Autodesk Inventor part; units mm, degrees
ref_plane "YZ Plane" through (0, 0, 0) normal (1, 0, 0) x (0, 1, 0)
ref_plane "XZ Plane" through (0, 0, 0) normal (0, 1, 0) x (-1, 0, 0)
ref_plane "XY Plane" through (0, 0, 0) normal (0, 0, 1) x (1, 0, 0)
sketch "Sketch1" plane through (0, 0, 0) normal (0, 1, 0) x (-1, 0, 0)
  arc A0 (0, -177) -> (0, 177) centre (0, 0) ccw
  arc A1 (0, 177) -> (0, -177) centre (0, 0) ccw
  point P0 (-177, 177)
  point P1 (-177, -177)
  dimension "d0" = 354
extrude "Extrusion1" add sketch "Sketch1" along normal blind 5
sketch "Sketch2" plane through (0, 5, 0) normal (0, 1, 0) x (1, 0, 0)
  circle A0 centre (-51.435, -34.125) radius 1.7
  circle A1 centre (-51.435, 34.125) radius 1.7
  circle A2 centre (51.435, 34.125) radius 1.7
  circle A3 centre (51.435, -34.125) radius 1.7
  line L0 (151.6, 177) -> (0, 177) construction
  line L1 (0, -177) -> (0, 177) construction
  circle A4 centre (0, 0) radius 177 construction
  line L2 (-177, 0) -> (177, 0) construction
  circle A5 centre (26.035, 59.5249) radius 1.7
  circle A6 centre (26.035, -59.5249) radius 1.7
  circle A7 centre (-26.035, 59.5249) radius 1.7
  circle A8 centre (-26.035, -59.5249) radius 1.7
  point P0 (177, 177)
  dimension "d5" = 3.4
  dimension "d6" = 3.4
  dimension "d8" = 3.4
  dimension "d10" = 3.4
  dimension "d12" = 68.25
  dimension "d13" = 68.25
  dimension "d14" = 102.87
  dimension "d15" = 102.87
  dimension "d18" = 51.435
  dimension "d19" = 51.435
  dimension "d20" = 34.125
  dimension "d21" = 34.125
  dimension "d153" = 3.4
  dimension "d155" = 3.4
  dimension "d157" = 3.4
  dimension "d159" = 3.4
  dimension "d161" = 52.07
  dimension "d162" = 26.035
  dimension "d163" = 52.07
  dimension "d164" = 26.035
  dimension "d165" = 119.0498
  dimension "d166" = 119.0498
  dimension "d167" = 59.5249
  dimension "d168" = 59.5249
extrude "Jetson Holes" cut sketch "Sketch2" against normal through all
sketch "Sketch3" plane through (0, 5, 0) normal (0, 1, 0) x (1, 0, 0)
  circle A0 centre (-12.7, -63.5) radius 9.525
  circle A1 centre (0, 0) radius 177 construction
  line L0 (151.6, 177) -> (0, 177) construction
  line L1 (-177, 0) -> (0, 0) construction
  line L2 (0, 0) -> (0, -177) construction
  point P0 (177, 177)
  dimension "d24" = 19.05
  dimension "d189" = 63.5
  dimension "d190" = 12.7
extrude "SPI_Holes" cut sketch "Sketch3" against normal through all
sketch "Sketch4" plane through (0, 5, 0) normal (0, 1, 0) x (1, 0, 0)
  circle A0 centre (-60.96, -76.2) radius 1.7
  circle A1 centre (60.96, -101.6) radius 1.7
  circle A2 centre (60.96, 76.2) radius 1.7
  circle A3 centre (-60.96, 101.6) radius 1.7
  line L0 (177, 0) -> (-177, 0) construction
  circle A4 centre (-12.7, -63.5) radius 9.525 construction
  circle A5 centre (-101.6, 50.8) radius 8.89
  circle A6 centre (-101.6, -50.8) radius 8.89
  circle A7 centre (41.91, -76.2) radius 1.7
  circle A8 centre (-41.91, -101.6) radius 1.7
  circle A9 centre (-41.91, 76.2) radius 1.7
  circle A10 centre (41.91, 101.6) radius 1.7
  point P0 (0, 0)
  point P1 (0, -177)
  dimension "d30" = 3.4
  dimension "d31" = 3.4
  dimension "d33" = 3.4
  dimension "d35" = 3.4
  dimension "d37" = 121.92
  dimension "d38" = 121.92
  dimension "d39" = 25.4
  dimension "d40" = 25.4
  dimension "d43" = 12.7
  dimension "d44" = 177.8
  dimension "d45" = 17.78
  dimension "d46" = 17.78
  dimension "d47" = 50.8
  dimension "d48" = 50.8
  dimension "d139" = 3.4
  dimension "d140" = 19.05
  dimension "d141" = 25.4
  dimension "d142" = 3.4
  dimension "d143" = 19.05
  dimension "d144" = 25.4
  dimension "d145" = 3.4
  dimension "d147" = 3.4
  dimension "d149" = 25.4
  dimension "d150" = 25.4
  dimension "d151" = 19.05
  dimension "d152" = 19.05
extrude "NiMH Holes" cut sketch "Sketch4" against normal through all
sketch "Sketch5" plane through (0, 5, 0) normal (0, 1, 0) x (1, 0, 0)
  circle A0 centre (-8.1625, 9.55) radius 1.7
  circle A1 centre (-8.1625, -9.55) radius 1.7
  circle A2 centre (8.1625, -9.55) radius 1.7
  circle A3 centre (8.1625, 9.55) radius 1.7
  line L0 (-177, 0) -> (177, 0)
  line L1 (0, 177) -> (0, -177) construction
  circle A4 centre (0, 0) radius 177 construction
  dimension "d53" = 3.4
  dimension "d54" = 3.4
  dimension "d56" = 3.4
  dimension "d58" = 3.4
  dimension "d60" = 16.325
  dimension "d61" = 16.325
  dimension "d62" = 19.1
  dimension "d63" = 19.1
  dimension "d66" = 9.55
  dimension "d67" = 9.55
  dimension "d191" = 8.1625
  dimension "d192" = 8.1625
extrude "IMU Holes" cut sketch "Sketch5" against normal through all
sketch "Sketch8" plane through (0, 5, 0) normal (0, 1, 0) x (1, 0, 0)
  circle A0 centre (-101.6, 101.6) radius 2.1907
  circle A1 centre (-101.6, -101.6) radius 2.1907
  circle A2 centre (101.6, -101.6) radius 2.1907
  circle A3 centre (101.6, 101.6) radius 2.1907
  line L0 (177, 0) -> (-177, 0) construction
  circle A4 centre (101.6, 0) radius 1.7
  point P0 (0, 0)
  dimension "d97" = 4.3815
  dimension "d98" = 4.3815
  dimension "d100" = 4.3815
  dimension "d102" = 4.3815
  dimension "d105" = 101.6
  dimension "d106" = 101.6
  dimension "d110" = 101.6
  dimension "d111" = 101.6
  dimension "d169" = 3.4
extrude "Level1 Standoffs" cut sketch "Sketch8" against normal through all
sketch "Sketch7" plane through (0, 5, 0) normal (0, 1, 0) x (1, 0, 0)
  line L0 (177, 0) -> (-177, 0) construction
  circle A0 centre (0, 0) radius 177 construction
  circle A1 centre (-141.44, 0) radius 2.667
  circle A2 centre (-114.4274, -83.1363) radius 2.667
  circle A3 centre (-114.4274, 83.1363) radius 2.667
  circle A4 centre (-43.7074, -134.5174) radius 2.667
  circle A5 centre (-43.7074, 134.5174) radius 2.667
  line L1 (0, 177) -> (0, -181.7127) construction
  circle A6 centre (141.44, 0) radius 2.667
  circle A7 centre (114.4274, -83.1363) radius 2.667
  circle A8 centre (114.4274, 83.1363) radius 2.667
  circle A9 centre (43.7074, -134.5174) radius 2.667
  circle A10 centre (43.7074, 134.5174) radius 2.667
  point P0 (-177, 0)
  point P1 (177, 0)
  dimension "d91" = 5.334
  dimension "d92" = 35.56
  dimension "d95" = 144
extrude "Zip Ties" cut sketch "Sketch7" against normal through all
sketch "Sketch12" plane through (0, 5, 0) normal (0, 1, 0) x (1, 0, 0)
  circle A0 centre (31.75, 63.5) radius 1.7
  circle A1 centre (-31.75, 63.5) radius 1.7
  circle A2 centre (-31.75, -63.5) radius 1.7
  circle A3 centre (31.75, -63.5) radius 1.7
  point P0 (0, 0)
  dimension "d193" = 3.4
  dimension "d194" = 3.4
  dimension "d195" = 3.4
  dimension "d196" = 3.4
  dimension "d197" = 63.5
  dimension "d198" = 63.5
  dimension "d199" = 63.5
  dimension "d200" = 63.5
  dimension "d201" = 31.75
  dimension "d202" = 31.75
  dimension "d203" = 31.75
  dimension "d204" = 31.75
extrude "LiDAR Standoffs" cut sketch "Sketch12" against normal blind 25.4
sketch "Sketch13" plane through (0, 5, 0) normal (0, 1, 0) x (1, 0, 0)
  circle A0 centre (-139.7, -17.145) radius 1.7
  circle A1 centre (-139.7, 17.145) radius 1.7
  point P0 (0, 0)
  dimension "d207" = 139.7
  dimension "d208" = 3.4
  dimension "d209" = 3.4
  dimension "d210" = 139.7
  dimension "d211" = 17.145
  dimension "d212" = 17.145
extrude "Astra Camera" cut sketch "Sketch13" against normal blind 25.4
equation "\"d0\" = robot_diameter"
equation "\"d3\" = hardboard_thickness"
equation "\"d5\" = m3_clearance"
equation "\"d6\" = d7"
equation "\"d8\" = d9"
equation "\"d10\" = d11"
equation "\"d13\" = d12"
equation "\"d19\" = d18"
equation "\"d20\" = d21"
equation "\"d21\" = 0.5 * d12"
equation "\"d153\" = d154"
equation "\"d155\" = d156"
equation "\"d157\" = d158"
equation "\"d159\" = d160"
equation "\"d162\" = 0.5 * d161"
equation "\"d163\" = d161"
equation "\"d164\" = d162"
equation "\"d166\" = d165"
equation "\"d167\" = 0.5 * d165"
equation "\"d168\" = d167"
equation "\"d30\" = m3_clearance"
equation "\"d31\" = d32"
equation "\"d33\" = d34"
equation "\"d35\" = d36"
equation "\"d38\" = d37"
equation "\"d40\" = d39"
equation "\"d46\" = d45"
equation "\"d48\" = d47"
equation "\"d139\" = m3_clearance"
equation "\"d141\" = d40"
equation "\"d142\" = m3_clearance"
equation "\"d144\" = d40"
equation "\"d145\" = d146"
equation "\"d147\" = d148"
equation "\"d149\" = d39"
equation "\"d150\" = d39"
equation "\"d152\" = d151"
equation "\"d53\" = m3_clearance"
equation "\"d54\" = d55"
equation "\"d56\" = d57"
equation "\"d58\" = d59"
equation "\"d61\" = d60"
equation "\"d63\" = d62"
equation "\"d66\" = 0.5 * d63"
equation "\"d67\" = d66"
equation "\"d106\" = d105"
equation "\"d110\" = d105"
equation "\"d111\" = d105"
equation "\"d169\" = m3_clearance"
equation "\"m3_heat_set_insert\" = 4"
equation "\"m3_clearance\" = 3.4"
equation "\"m3_heat_set_depth\" = 7"
equation "\"robot_diameter\" = 354"
equation "\"hardboard_thickness\" = 5"
equation "\"motor_centerline_height\" = 13"
properties part number "layer2_short"
Read the model definition and answer for the solid it produces. Units are mm, in the model's axes. Give positions to 0.01 mm unless a question says otherwise; leave off trailing zeros. Write each loop counter-clockwise with the first axis right and the second up, starting at its lowest first coordinate (ties: lowest second). Pieces come first, ordered by that corner, then holes. Notation, with made-up numbers: M -32.5,76.5 L 11.5,76.5 A14 ccw 11.5,89.5 Z; hole C 13.5,-6.75 d7. An arc over 180 degrees is marked long. Put each result on its own line as item: value. Start each with the question number.
1. The part is cut by section B-B, the plane y = 2.65. Give the number of separate pieces and of enclosed holes in the cut face, and give its area (3 significant figures).
2. Each of these flat-tipped pins is pushed along its axis until it touches: pin 1 Ø4.5 at (x, z) = (-26.04, -59.52) entering from +Y; pin 2 Ø3.5 at (x, z) = (-101.6, -101.6) entering from +Y; pin 3 Ø2 at (x, y) = (79.5, 1.5) entering from +Z; pin 4 Ø2 at (x, y) = (68, 2) entering from -Z. Where does it stop, or does it pass through?
3. The part is cut by section A-A, the plane z = -93. Give the vertices of the cut face in (x, y).
4. For a pull along X with two mould halves and no side action, classify faces 1 (the cylindrical face through (-110.48, 2.54, -51.19)), 2 (the cylindrical face through (172.79, 2.46, -38.37)), 3 (the flat face through (2, 0, 2)) as released by +X, released by -X, zero draft, split by the parting line, or undercut.
5. Consider line 1 along Z through (x, y) = (101.6, 3.3); line 2 along Z through (x, y) = (9.5, 1.3); line 3 along X through (y, z) = (4.4, -8). Determine where each line is inside the solid, lowest interval first.
6. The part is cut by section C-C, the plane z = -153. Give the vertices of the cut face in (x, y), and give its area (3 significant figures).
Final values:
1. separate pieces: 1
1. enclosed holes: 44
1. area: 97,100 mm²
2. pin 1: stops at y = 5
2. pin 2: passes through
2. pin 3: stops at z = 158.64
2. pin 4: stops at z = -163.83
3. outline: M -150.6,0 L 150.6,0 L 150.6,5 L -150.6,5 Z
4. face 1: undercut
4. face 2: split by the parting line
4. face 3: zero draft
5. line 1: z = -144.94 to -103.79, -99.41 to -1.7, 1.7 to 99.41, 103.79 to 144.94
5. line 2: z = -176.74 to -10.6, -8.5 to 8.5, 10.6 to 176.74
5. line 3: x = -176.82 to -8.86, -7.46 to 7.46, 8.86 to 176.82
6. outline: M -88.99,0 L 88.99,0 L 88.99,5 L -88.99,5 Z
6. area: 890 mm²
